```python
from build123d import *
from build123d.topology import SkipClean

# Parameters (mm, degrees)
BOSS_EXTRUDE1_DEPTH                           = 2.54
BOSS_EXTRUDE2_DEPTH                           = 2.54
FILLET1_R                                     = 2.286
CBORE_FOR_4_BUTTON_HEAD_CAP_SCREW_D           = 3.2639
CBORE_FOR_4_BUTTON_HEAD_CAP_SCREW_CBORE_D     = 6.35
CBORE_FOR_4_BUTTON_HEAD_CAP_SCREW_CBORE_DEPTH = 1.4986
SKETCH6_W                                     = 14.4
SKETCH6_H                                     = 25.7
CUT_EXTRUDE1_DEPTH                            = 244.87875068
SKETCH7_W                                     = 19.48
SKETCH7_H                                     = 30.78
CUT_EXTRUDE2_DEPTH                            = 1.27
CHAMFER1_SIZE                                 = 1
F_4_40_TAPPED_HOLE1_D                         = 2.2606
F_4_40_TAPPED_HOLE1_DEPTH                     = 1.27
F_4_40_TAPPED_HOLE1_TIP                       = 0.679152758
BOSS_EXTRUDE3_START                           = -2
BOSS_EXTRUDE3_OUTLINE_R                       = 1.85
BOSS_EXTRUDE3_OUTLINE_R_2                     = 1.1303
BOSS_EXTRUDE3_DEPTH                           = 3.397
CHAMFER2_SIZE                                 = 1


with BuildPart() as part:
    # Sketch1 → Boss-Extrude1 (new body)
    with BuildSketch(Plane(origin=(0, 0, 0), x_dir=(1, 0, 0), z_dir=(0, 1, 0))):
        with BuildLine():
            Line((24.13, 24.13), (-26.67, 24.13))
            ThreePointArc((-26.67, 24.13), (-28.466051224, 23.386051224), (-29.21, 21.59))
            Line((-29.21, 21.59), (-29.21, -21.59))
            ThreePointArc((-29.21, -21.59), (-28.466051224, -23.386051224), (-26.67, -24.13))
            Line((-26.67, -24.13), (24.13, -24.13))
            ThreePointArc((24.13, -24.13), (25.926051224, -23.386051224), (26.67, -21.59))
            Line((26.67, -21.59), (26.67, 21.59))
            ThreePointArc((26.67, 21.59), (25.926051224, 23.386051224), (24.13, 24.13))
        make_face()
    extrude(amount=BOSS_EXTRUDE1_DEPTH)

    # Sketch3 → Boss-Extrude2 (add)
    with BuildSketch(Plane.XZ):
        with BuildLine():
            Line((24.638, -21.59), (24.638, 21.59))
            ThreePointArc((24.638, 21.59), (24.489210245, 21.949210245), (24.13, 22.098))
            Line((24.13, 22.098), (-26.67, 22.098))
            ThreePointArc((-26.67, 22.098), (-27.029210245, 21.949210245), (-27.178, 21.59))
            Line((-27.178, 21.59), (-27.178, -21.59))
            ThreePointArc((-27.178, -21.59), (-27.029210245, -21.949210245), (-26.67, -22.098))
            Line((-26.67, -22.098), (24.13, -22.098))
            ThreePointArc((24.13, -22.098), (24.489210245, -21.949210245), (24.638, -21.59))
        make_face()
        with BuildLine():
            Line((-20.881289338, -20.193), (18.341289338, -20.193))
            ThreePointArc((18.341289338, -20.193), (19.403923164, -16.863923164), (22.733, -15.801289338))
            Line((22.733, -15.801289338), (22.733, 15.801289338))
            ThreePointArc((22.733, 15.801289338), (19.403923164, 16.863923164), (18.341289338, 20.193))
            Line((18.341289338, 20.193), (-20.881289338, 20.193))
            ThreePointArc((-20.881289338, 20.193), (-21.943923164, 16.863923164), (-25.273, 15.801289338))
            Line((-25.273, 15.801289338), (-25.273, -15.801289338))
            ThreePointArc((-25.273, -15.801289338), (-21.943923164, -16.863923164), (-20.881289338, -20.193))
        make_face(mode=Mode.SUBTRACT)
    extrude(amount=BOSS_EXTRUDE2_DEPTH)

    # Fillet1
    fillet1_edges = [part.edges().sort_by_distance(p)[0] for p in [
        (-28.466051224, 2.54, -23.386051224),
        (-29.21, 2.54, 0),
        (-28.466051224, 2.54, 23.386051224),
        (-1.27, 2.54, 24.13),
        (25.926051224, 2.54, 23.386051224),
        (26.67, 2.54, 0),
        (25.926051224, 2.54, -23.386051224),
        (-1.27, 2.54, -24.13),
    ]]
    fillet(fillet1_edges, radius=FILLET1_R)

    # CBORE for #4 Button Head Cap Screw (through all)
    with Locations(Plane(origin=(107.325337048, 2.54, -177.882723122), x_dir=(1, 0, 0), z_dir=(0, 1, 0))):
        with Locations((-85.735337048, -158.832723122), (-85.735337048, -196.932723122), (-131.455337048, -158.832723122), (-131.455337048, -196.932723122)):
            CounterBoreHole(CBORE_FOR_4_BUTTON_HEAD_CAP_SCREW_D / 2, CBORE_FOR_4_BUTTON_HEAD_CAP_SCREW_CBORE_D / 2, CBORE_FOR_4_BUTTON_HEAD_CAP_SCREW_CBORE_DEPTH)

    # Sketch6 → Cut-Extrude1 (cut, through all)
    with BuildSketch(Plane(origin=(107.325337048, 2.54, -177.882723122), x_dir=(-1, 0, 0), z_dir=(0, 1, 0))):
        with Locations((98.306283227, 177.882723122)):
            Rectangle(SKETCH6_W, SKETCH6_H)
    extrude(amount=-CUT_EXTRUDE1_DEPTH, mode=Mode.SUBTRACT)

    # Sketch7 → Cut-Extrude2 (cut)
    with BuildSketch(Plane.XZ):
        with Locations((9.019053821, 0)):
            Rectangle(SKETCH7_W, SKETCH7_H)
    extrude(amount=-CUT_EXTRUDE2_DEPTH, mode=Mode.SUBTRACT)

    # Chamfer1
    chamfer1_edges = [part.edges().sort_by_distance(p)[0] for p in [
        (16.219053821, 2.54, 0),
        (9.019053821, 2.54, -12.85),
        (1.819053821, 2.54, 0),
        (9.019053821, 2.54, 12.85),
    ]]
    chamfer(chamfer1_edges, length=CHAMFER1_SIZE)

    # #4-40 Tapped Hole1
    with Locations(Plane(origin=(107.325337048, 0, -177.882723122), x_dir=(-1, 0, 0), z_dir=(0, -1, 0))):
        with Locations((88.486283227, -189.532723122), (88.486283227, -166.232723122), (112.286283227, -166.232723122), (112.286283227, -189.532723122)):
            Hole(F_4_40_TAPPED_HOLE1_D / 2, depth=F_4_40_TAPPED_HOLE1_DEPTH)
            with Locations((0, 0, -(F_4_40_TAPPED_HOLE1_DEPTH + F_4_40_TAPPED_HOLE1_TIP / 2))):  # 118° drill point
                Cone(0, F_4_40_TAPPED_HOLE1_D / 2, F_4_40_TAPPED_HOLE1_TIP, mode=Mode.SUBTRACT)

    # Boss-Extrude3: read off the stored shape, not the designer's step
    # Boss-Extrude3 outline → Boss-Extrude3 (add)
    # profile 1 of 4: a face of its own
    with SkipClean():  # the faces are left unmerged after this step: merging them gives an invalid solid
        with BuildSketch(Plane.XZ.offset(BOSS_EXTRUDE3_START)):
            with Locations((18.839053821, 11.65)):
                Circle(BOSS_EXTRUDE3_OUTLINE_R)
            with Locations((18.839053821, 11.65)):
                Circle(BOSS_EXTRUDE3_OUTLINE_R_2, mode=Mode.SUBTRACT)
        # profile 2 of 4: a face of its own
        with BuildSketch(Plane.XZ.offset(BOSS_EXTRUDE3_START)):
            with Locations((18.839053821, -11.65)):
                Circle(BOSS_EXTRUDE3_OUTLINE_R)
            with Locations((18.839053821, -11.65)):
                Circle(BOSS_EXTRUDE3_OUTLINE_R_2, mode=Mode.SUBTRACT)
        # profile 3 of 4: a face of its own
        with BuildSketch(Plane.XZ.offset(BOSS_EXTRUDE3_START)):
            with Locations((-4.960946179, -11.65)):
                Circle(BOSS_EXTRUDE3_OUTLINE_R)
            with Locations((-4.960946179, -11.65)):
                Circle(BOSS_EXTRUDE3_OUTLINE_R_2, mode=Mode.SUBTRACT)
        # profile 4 of 4: a face of its own
        with BuildSketch(Plane.XZ.offset(BOSS_EXTRUDE3_START)):
            with Locations((-4.960946179, 11.65)):
                Circle(BOSS_EXTRUDE3_OUTLINE_R)
            with Locations((-4.960946179, 11.65)):
                Circle(BOSS_EXTRUDE3_OUTLINE_R_2, mode=Mode.SUBTRACT)
        extrude(amount=BOSS_EXTRUDE3_DEPTH)

    # Chamfer2
    chamfer2_edges = [part.edges().sort_by_distance(p)[0] for p in [
        (20.118604523, 0, 10.313867522),
        (20.118604523, 0, -12.986132478),
        (-6.810946179, 0, -11.65),
        (-6.810946179, 0, 11.65),
    ]]
    chamfer(chamfer2_edges, length=CHAMFER2_SIZE)


solid = part.part
```
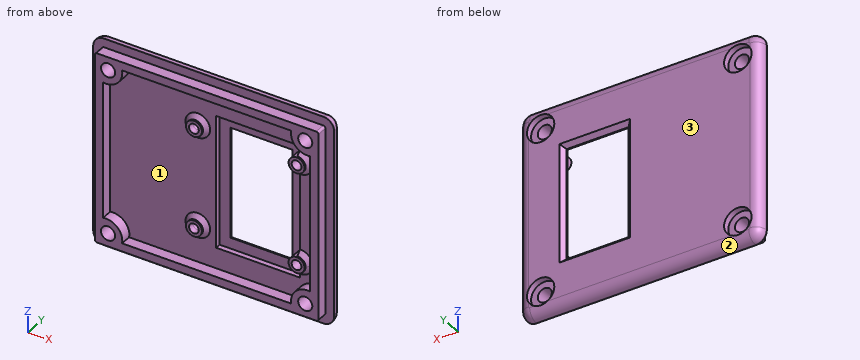
The listing builds one solid part. Answer for the finished solid, in the listing's coordinates (mm). Face numbers are marked on the shaded views. Round coordinates to 2 decimals unless told otherwise and drop trailing zeros. Order: outer loops, then holes, each group sorted by start corner. A loop starts at its lowest first (then second) coordinate and runs counter-clockwise, first axis right, second up. Notation, with made-up numbers: (2, 53.25) -> (32, 53.25) arc R26 cw to (32, 73.25) -> close; hole circle Ø2 at (51, 30.25). An arc over 180 degrees is marked (long way). Answer as CSV lines item,"result". Start each with the question number.
(1) Flat-ended cylindrical pins translate along their axes: pin 1 Ø1.3 at (x, y) = (-11, -1.5) entering from +Z; pin 2 Ø1.3 at (y, z) = (-1.5, 5.5) entering from +X; pin 3 Ø1 at (x, y) = (10, 1) entering from -Z. Find the tip coordinate at first contact, or state that the pin passes through.
(2) The part is cut by section D-D (z = 19.05). Determine the outline of the cut face in (x, y) (3 decimals), then the cut area to 3 significant figures.
(3) The part is cut by section B-B (x = 10). Determine the outline of the cut face in (y, z).
(4) For a pull along Z with two mould halves and no side action, classify the marked faces 1, 2 and 3 as +Z half, -Z half, draft (parallel to the pull), parting line (faces both ways), or undercut.
(5) The part is cut by section C-C (x = -24.13). Determine the outline of the cut face in (y, z) (3 decimals).
(6) The part is cut by section A-A (z = -7). Determine the outline of the cut face in (x, y), then the cut area to 3 significant figures.
(7) Find the intervals of material crossed by probe 1 along Z at (x, y) = (12, -2.3); probe 2 along X at (y, z) = (0.1, -8.5); probe 3 along Z at (x, y) = (21.59, 1.45) (3 decimals), in increasing order. Write a range as from..to.
Evaluation:
1,pin 1,"z = 22.1"
1,pin 2,"x = 24.64"
1,pin 3,"z = -24.12"
2,outline,"(-29.21, 0) -> (-27.178, 0) -> (-27.178, -2.54) -> (-25.762, -2.54) -> (-25.762, 1.041) -> (-27.305, 1.041) -> (-27.305, 2.508) arc R2.286 ccw to (-29.21, 0.254) -> close; (-22.498, -2.54) -> (-20.862, -2.54) -> (-20.862, 0) -> (18.322, 0) -> (18.322, -2.54) -> (19.958, -2.54) -> (19.958, 1.041) -> (18.415, 1.041) -> (18.415, 2.54) -> (-20.955, 2.54) -> (-20.955, 1.041) -> (-22.498, 1.041) -> close; (23.222, -2.54) -> (24.638, -2.54) -> (24.638, 0) -> (26.67, 0) -> (26.67, 0.254) arc R2.286 ccw to (24.765, 2.508) -> (24.765, 1.041) -> (23.222, 1.041) -> close"
2,area,"129 mm²"
3,outline,"(-2.54, -22.1) -> (0, -22.1) -> (0, -24.13) -> (0.25, -24.13) arc R2.29 ccw to (2.54, -21.84) -> (2.54, -13.85) -> (1.54, -12.85) -> (1.27, -12.85) -> (1.27, -15.39) -> (0, -15.39) -> (0, -20.19) -> (-2.54, -20.19) -> close; (-2.54, 20.19) -> (0, 20.19) -> (0, 15.39) -> (1.27, 15.39) -> (1.27, 12.85) -> (1.54, 12.85) -> (2.54, 13.85) -> (2.54, 21.84) arc R2.29 ccw to (0.25, 24.13) -> (0, 24.13) -> (0, 22.1) -> (-2.54, 22.1) -> close"
4,face 1,"undercut"
4,face 2,"-Z half"
4,face 3,"draft"
5,outline,"(-2.54, -22.098) -> (0, -22.098) -> (0, -24.13) -> (0.254, -24.13) arc R2.286 ccw to (2.508, -22.225) -> (1.041, -22.225) -> (1.041, -20.682) -> (-2.54, -20.682) -> close; (-2.54, -17.418) -> (1.041, -17.418) -> (1.041, -15.875) -> (2.54, -15.875) -> (2.54, 15.875) -> (1.041, 15.875) -> (1.041, 17.418) -> (-2.54, 17.418) -> (-2.54, 15.782) -> (0, 15.782) -> (0, -15.782) -> (-2.54, -15.782) -> close; (-2.54, 20.682) -> (1.041, 20.682) -> (1.041, 22.225) -> (2.508, 22.225) arc R2.286 ccw to (0.254, 24.13) -> (0, 24.13) -> (0, 22.098) -> (-2.54, 22.098) -> close"
6,outline,"(-29.21, 0) -> (-27.18, 0) -> (-27.18, -2.54) -> (-25.27, -2.54) -> (-25.27, 0) -> (-0.72, 0) -> (-0.72, 1.27) -> (1.82, 1.27) -> (1.82, 1.54) -> (0.82, 2.54) -> (-26.92, 2.54) arc R2.29 ccw to (-29.21, 0.25) -> close; (16.22, 1.27) -> (18.76, 1.27) -> (18.76, 0) -> (22.73, 0) -> (22.73, -2.54) -> (24.64, -2.54) -> (24.64, 0) -> (26.67, 0) -> (26.67, 0.25) arc R2.29 ccw to (24.38, 2.54) -> (17.22, 2.54) -> (16.22, 1.54) -> close"
6,area,"105 mm²"
7,probe 1,"-22.1..-20.19, 20.19..22.1"
7,probe 2,"-29.21..-0.72, 18.76..26.67"
7,probe 3,"-23.792..-22.225, -15.875..15.875, 22.225..23.792"
